from build123d import *

# Parameters (mm, degrees)
F1_DEPTH = 3.175
F2_R     = 3.81
F3_DEPTH = 25.4


with BuildPart() as f1:
    # F0 (on Top) → F1 (new body)
    with BuildSketch(Plane.XY):
        with BuildLine():
            Line((-515.62, 0), (0, 0))
            Line((0, 0), (515.62, 0))
            Line((515.62, 0), (520.7, 0))
            Line((520.7, 0), (520.7, 5.08))
            Line((520.7, 5.08), (520.7, 175.961931))
            ThreePointArc((520.7, 175.961931), (513.495857, 198.256685), (494.60782, 212.120226))
            ThreePointArc((494.60782, 212.120226), (0, 292.1), (-494.60782, 212.120226))
            ThreePointArc((-494.60782, 212.120226), (-513.495857, 198.256685), (-520.7, 175.961931))
            Line((-520.7, 175.961931), (-520.7, 5.08))
            Line((-520.7, 5.08), (-520.7, 0))
            Line((-520.7, 0), (-515.62, 0))
        make_face()
    extrude(amount=F1_DEPTH)

    # F2 (on face) → F3 (cut)
    with BuildSketch(Plane.XY.offset(3.175)):
        with Locations((510.54, 10.16)):
            Circle(F2_R)
        with Locations((368.3, 10.16)):
            Circle(F2_R)
        with Locations((226.06, 10.16)):
            Circle(F2_R)
        with Locations((-226.06, 10.16)):
            Circle(F2_R)
        with Locations((-368.3, 10.16)):
            Circle(F2_R)
        with Locations((-510.54, 10.16)):
            Circle(F2_R)
    extrude(amount=-F3_DEPTH, mode=Mode.SUBTRACT)


solid = f1.part
The listing builds one solid part. Answer for the finished solid, in the listing's coordinates (mm). Round coordinates to 2 decimals unless told otherwise and drop trailing zeros. Order: outer loops, then holes, each group sorted by start corner. A loop starts at its lowest first (then second) coordinate and runs counter-clockwise, first axis right, second up. Notation, with made-up numbers: (-11, -13.5) -> (17, -13.5) arc R17 ccw to (17, 17.5) -> close; hole circle Ø6 at (-40, 29.25). An arc over 180 degrees is marked (long way). Put each result on its own line as item: value.
Q1. Consider line 1 along Y through (x, z) = (-510.54, 0.95); line 2 along Y through (x, z) = (368.3, 2); line 3 along X through (y, z) = (178, 2.1). Determine where each line is inside the solid, lowest interval first.
Results list:
line 1: 0 to 6.35, 13.97 to 201.86
line 2: 0 to 6.35, 13.97 to 248.27
line 3: -520.65 to 520.65
Q2. Section C-C, the plane y = 249.5 is taken. Write down the section's boundary in (x, z) (3 decimals), and give its area (3 significant figures).
Results list:
outline: (-363.173, 0) -> (363.173, 0) -> (363.173, 3.175) -> (-363.173, 3.175) -> close
area: 2,310 mm^2
Q3. This flat-tipped pin is pushed along its axis until it touches: P1, Ø4.5, axis at x = -226.06, y = 10.16, coming from the -Z side. Where does it stop, or does it pass through?
Results list:
P1: through
Q4. Section A-A, the plane z = 2.1 is taken. Write down the section's boundary in (x, y), and give its area (3 significant figures).
Results list:
outline: (-520.7, 0) -> (520.7, 0) -> (520.7, 175.96) arc R38.1 ccw to (494.61, 212.12) arc R1569.36 ccw to (-494.61, 212.12) arc R38.1 ccw to (-520.7, 175.96) -> close; hole circle Ø7.62 at (-510.54, 10.16); hole circle Ø7.62 at (-368.3, 10.16); hole circle Ø7.62 at (-226.06, 10.16); hole circle Ø7.62 at (226.06, 10.16); hole circle Ø7.62 at (368.3, 10.16); hole circle Ø7.62 at (510.54, 10.16)
area: 273,000 mm^2
Q5. Section B-B, the plane x = -424.5 is taken. Write down the section's boundary in (y, z) (3 decimals).
Results list:
outline: (0, 0) -> (233.597, 0) -> (233.597, 3.175) -> (0, 3.175) -> close
